Here's how the part is built. I have some questions about the finished solid (model axes, mm). A direction names the side the tool comes from. Coordinates: 2 decimals unless noted, no trailing zeros. Write each loop counter-clockwise with the first axis right and the second up, starting at its lowest first coordinate (ties: lowest second). Pieces come first, ordered by that corner, then holes.
Item 1: If we section it at A-A (z = 4.5): Count the separate pieces of the cut face and the enclosed holes in it, then the cut area to 3 significant figures.
Item 2: I'm going to push flat-ended pins straight in: pin 1 Ø4 at (y, z) = (3, 6.5) entering from -X; pin 2 Ø6.5 at (y, z) = (6, 6) entering from -X (3 decimals); pin 3 Ø5.5 at (x, z) = (-14.29, 6) entering from +Y; pin 4 Ø3.5 at (x, z) = (-14.29, 6) entering from +Y. Where does each tip first touch, or does it pass through?
Item 3: If we section it at B-B (x = -26.25): Please give me the cut outline in (y, z), then the cut area to 3 significant figures.
Item 4: For faces 4 (the face through (-0.901, 3.356, 6.084)), 5 (the face through (-17.983, 11.499, 4.468)), 6 (the face through (-11, 5.746, 2)), which set-ups out of +Z, -Z, +X, -X, +Y, -Y let a thin tool reach every point of the face, with its end or its side?
Item 5: If I drill on line 1 (Z direction, x = -27.9, y = 6); line 2 (Y direction, x = -20.25, z = 11.25); line 3 (X direction, y = 11.5, z = 4.5), over which ranges is the centre line in solid material (lowest first)?
Item 6: If we section it at C-C (z = 8.5): Please give me the cut outline in (x, y) (3 decimals).
Item 7: We'd pull the mould along Z, two halves only. Please class faces 1 (the face through (-0.43, 11.55, 5.92)), 2 (the face through (-12.232, 9.178, 6.09)), 3 (the face through (-11, 7, 12)): +Z half, -Z half, draft (parallel to the pull), parting line (faces both ways), or undercut.
from build123d import *

# Parameters (mm, degrees)
F1_DEPTH = 12
F2_R     = 2.0574
F3_DEPTH = 12.001
F4_R     = 4.0005
F5_DEPTH = 1.016
F6_R     = 2
F7_DEPTH = 28.576
F9_DEPTH = 12.001


with BuildPart() as f1:
    # F0 (on Top) → F1 (new body)
    with BuildSketch(Plane.XY):
        with BuildLine():
            Line((-22.575, 0), (-1.5, 0))
            ThreePointArc((-1.5, 0), (-0.43934, 0.43934), (0, 1.5))
            Line((0, 1.5), (0, 5.746))
            Line((0, 5.746), (-21.219176, 5.746))
            ThreePointArc((-21.219176, 5.746), (-27.559, 6), (-21.219176, 6.254))
            Line((-21.219176, 6.254), (0, 6.254))
            Line((0, 6.254), (0, 10.5))
            ThreePointArc((0, 10.5), (-0.43934, 11.56066), (-1.5, 12))
            Line((-1.5, 12), (-22.575, 12))
            ThreePointArc((-22.575, 12), (-28.575, 6), (-22.575, 0))
        make_face()
    extrude(amount=F1_DEPTH)

    # F2 (on face) → F3 (cut, through all)
    with BuildSketch(Plane(origin=(0, 12, 0), x_dir=(-1, 0, 0), z_dir=(0, 1, 0))):
        with Locations((14.2875, 6)):
            Circle(F2_R)
    extrude(amount=-F3_DEPTH, mode=Mode.SUBTRACT)

    # F4 (on face) → F5 (cut)
    with BuildSketch(Plane(origin=(0, 12, 0), x_dir=(-1, 0, 0), z_dir=(0, 1, 0))):
        with Locations((14.2875, 6)):
            Circle(F4_R)
    extrude(amount=-F5_DEPTH, mode=Mode.SUBTRACT)

    # F6 (on face) → F7 (cut, through all)
    with BuildSketch(Plane.YZ):
        with Locations((6, 6)):
            Circle(F6_R)
    extrude(amount=-F7_DEPTH, mode=Mode.SUBTRACT)

    # F8 (on face) → F9 (cut, through all)
    with BuildSketch(Plane.XY.offset(12)):
        Polygon((0, 6.254), (0, 8.123071), (-1.778, 9.1496), (-1.778, 2.8504), (0, 3.876929), (0, 5.746), align=None)
    extrude(amount=-F9_DEPTH, mode=Mode.SUBTRACT)


solid = f1.part
Answer list:
1. separate pieces: 4
1. enclosed holes: 0
1. area: 200 mm2
2. pin 1: stops at x = -28.44
2. pin 2: stops at x = -28.575
2. pin 3: stops at y = 10.98
2. pin 4: passes through
3. outline: (1.26, 0) - (3.43, 0) - (3.43, 12) - (1.26, 12) - close; (8.57, 0) - (10.74, 0) - (10.74, 12) - (8.57, 12) - close
3. area: 52.2 mm2
4. face 4: +Z, -Z
4. face 5: +Y
4. face 6: +Z, -Z, +X
5. line 1: z = 0 to 4, 8 to 12
5. line 2: y = 0 to 5.75, 6.25 to 12
5. line 3: x = -24.97 to -18, -10.58 to -0.38
6. outline: (-22.575, 0) - (-1.5, 0) arc R1.5 ccw to (0, 1.5) - (0, 3.877) - (-1.778, 2.85) - (-1.778, 5.746) - (-21.219, 5.746) arc R3.175 cw (long way) to (-21.219, 6.254) - (-1.778, 6.254) - (-1.778, 9.15) - (0, 8.123) - (0, 10.5) arc R1.5 ccw to (-1.5, 12) - (-11.164, 12) - (-11.164, 10.984) - (-17.411, 10.984) - (-17.411, 12) - (-22.575, 12) arc R6 ccw to start
7. face 1: draft
7. face 2: undercut
7. face 3: +Z half
